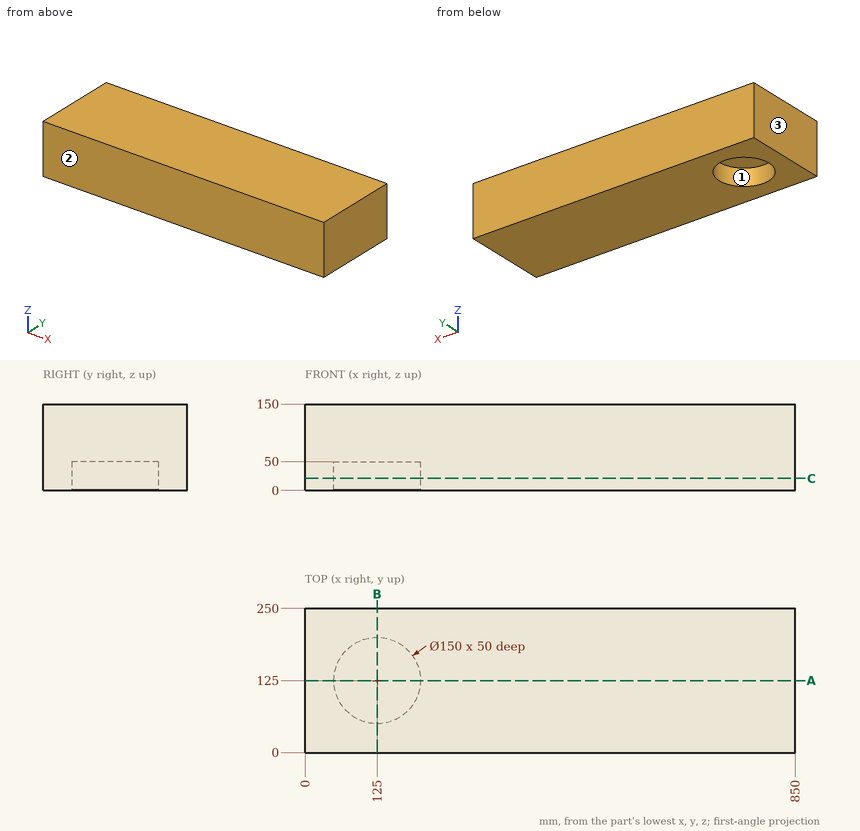
Part print with two shaded views. Sizes in mm from the minimum x, y, z corner. Round coordinates to 2 decimals unless told otherwise and drop trailing zeros. Loops run counter-clockwise (first coordinate to the right, second up) from the corner with the lowest first, then second, coordinate; pieces in that order, holes last. Notation, with made-up numbers: M 30.25,18 L 72.25,18 A21 cw 72.25,44 Z; hole C -18,1.25 d5. An arc over 180 degrees is marked long. Return JSON: item names as keys, results as strings. Group by question number.
(1) Saw through at A-A, the plane y = 125. List the corners of the cut face in (x, z).
(2) Wall check: probe 1 along Y at (x, z) = (125, 21); probe 2 along Z at (x, y) = (167, 95.5); probe 3 along X at (y, z) = (64, 36). Give the ranges that are in metal, low to high. Write a range as [from, to].
(3) Saw through at B-B, the plane x = 125. List the corners of the cut face in (y, z).
(4) Mould opens along X. For the marked faces 1, 2 and 3 say: +X half, -X half, draft (parallel to the pull), parting line (faces both ways), or undercut.
(5) Saw through at C-C, the plane z = 21. List the corners of the cut face in (x, y), and give its area (3 significant figures).
Answer list:
{
 "1": {"outline": "M 0,0 L 50,0 L 50,50 L 200,50 L 200,0 L 850,0 L 850,150 L 0,150 Z"},
 "2": {"probe 1": "[0, 50], [200, 250]", "probe 2": "[50, 150]", "probe 3": "[0, 81.37], [168.63, 850]"},
 "3": {"outline": "M 0,0 L 50,0 L 50,50 L 200,50 L 200,0 L 250,0 L 250,150 L 0,150 Z"},
 "4": {"face 1": "undercut", "face 2": "draft", "face 3": "-X half"},
 "5": {"outline": "M 0,0 L 850,0 L 850,250 L 0,250 Z; hole C 125,125 d150", "area": "195,000 mm2"}
}
